Source: CAD feature listing. Evaluate the final solid. Frame: model axes, mm. A direction names the side the tool comes from. Round coordinates to 2 decimals unless told otherwise and drop trailing zeros. Order: outer loops, then holes, each group sorted by start corner. A loop starts at its lowest first (then second) coordinate and runs counter-clockwise, first axis right, second up. Notation, with made-up numbers: (-8, -18) -> (34, -18) arc R18 ccw to (34, -1) -> close; hole circle Ø4 at (-19, 62). An arc over 180 degrees is marked (long way). Answer as CSV lines item,"result". Start each with the question number.
(1) Line query: line 1 along Z through (x, y) = (0, -0.7) (3 decimals); line 2 along Z through (x, y) = (0, 8.95); line 3 along X through (y, z) = (4.5, -0.5). Output: solid intervals per line, ascending. Write a range as from..to.
(2) Section query C-C (y = 8). Output: boundary loops of the cut face in (x, z), plus the area to 3 significant figures.
(3) Section query A-A (x = 0). Output: boundary loops of the cut face in (y, z) (3 decimals), plus the area to 3 significant figures.
(4) Contact query for flat-ended pins moving along their axis: P1, Ø1.8, axis at x = -0.5, z = 0.5, coming from the +Y side; P2, Ø4, axis at y = 2, z = -2.5, coming from the -X side; P3, Ø2.5, axis at x = 0, z = -0.5, coming from the -Y side; P4, Ø2, axis at y = 6, z = 3, coming from the +X side. Output: stop coordinate, or through.
(5) Pull-direction query (Z, two-part tool) for faces 1 (the conical face through (2.924, 2.864, -0.921)), 2 (the flat face through (2, 6.57, -1)), 3 (the flat face through (-3, 7.5, 1)); classes: +Z half, -Z half, draft (parallel to the pull), parting line (faces both ways), or undercut.
(6) Set-up query: faces 4 (the conical face through (-1.712, 3.084, 1.313)), 5 (the cylindrical face through (-0.31, -0.868, 2.365)), 6 (the cylindrical face through (0.39, 8.14, -1.74)). Return all of +Z, -Z, +X, -X, +Y, -Y with unobstructed straight access to the full face (end or side cutting, diameter ignored); none if empty.
(7) Section query B-B (y = -0.25). Output: boundary loops of the cut face in (x, z) (3 decimals).
```python
from build123d import *

# Parameters (mm, degrees)
F0_R       = 3.765
F1_DEPTH   = 7.5
F1_FACE1_R = 3.765
F2_R       = 2.6326071787
F4_R       = 2.385
F5_DEPTH   = 1.76
F6_R       = 2.7120257238
F7_DEPTH   = 2.25
F8_T       = -0.93


with BuildPart() as f1:
    # F0 (on Front) → F1 (new body)
    with BuildSketch(Plane.XZ):
        Circle(F0_R)
    extrude(amount=-F1_DEPTH)

    # F1_face1 (on face) → F3 section 0
    with BuildSketch(Plane(origin=(0, 7.5, 0), x_dir=(1, 0, 0), z_dir=(0, 1, 0))):
        Circle(F1_FACE1_R)
    # F2 (on face) → F3 section 1
    with BuildSketch(Plane.XZ):
        Circle(F2_R)
    loft(mode=Mode.INTERSECT)

    # F4 (on Front) → F5 (join)
    with BuildSketch(Plane.XZ):
        Circle(F4_R)
    extrude(amount=F5_DEPTH)

    # F6 (on face) → F7 (join)
    with BuildSketch(Plane(origin=(0, 7.5, 0), x_dir=(-1, 0, 0), z_dir=(0, 1, 0))):
        Circle(F6_R)
    extrude(amount=F7_DEPTH)

    # F8
    f8_openings = [f1.faces().sort_by_distance(p)[0] for p in [
        (0, -1.76, 0),
        (0, 9.75, 0),
    ]]
    offset(amount=F8_T, openings=f8_openings, kind=Kind.INTERSECTION)


solid = f1.part
```
Answer block:
1,line 1,"-2.385..-1.455, 1.455..2.385"
1,line 2,"-2.71..-1.78, 1.78..2.71"
1,line 3,"-3.27..-2.32, 2.32..3.27"
2,outline,"circle Ø5.42 at (0, 0); hole circle Ø3.56 at (0, 0)"
2,area,"13.1 mm2"
3,outline,"(-1.76, -2.385) -> (0, -2.385) -> (0, -2.633) -> (7.5, -3.765) -> (7.5, -2.712) -> (9.75, -2.712) -> (9.75, -1.782) -> (6.57, -1.782) -> (6.57, -2.684) -> (0.93, -1.832) -> (0.93, -1.455) -> (-1.76, -1.455) -> close; (-1.76, 1.455) -> (0.93, 1.455) -> (0.93, 1.832) -> (6.57, 2.684) -> (6.57, 1.782) -> (9.75, 1.782) -> (9.75, 2.712) -> (7.5, 2.712) -> (7.5, 3.765) -> (0, 2.633) -> (0, 2.385) -> (-1.76, 2.385) -> close"
3,area,"23.9 mm2"
4,P1,"y = 0.93"
4,P2,"x = -2.99"
4,P3,"y = -1.76"
4,P4,"x = 2.94"
5,face 1,"parting line"
5,face 2,"undercut"
5,face 3,"draft"
6,face 4,"none"
6,face 5,"-Y"
6,face 6,"+Y"
7,outline,"circle Ø4.77 at (0, 0); hole circle Ø2.91 at (0, 0)"
